from build123d import *

# Parameters (mm, degrees)
SKETCH1_R           = 1.6
BOSS_EXTRUDE1_DEPTH = 6
CUT_EXTRUDE1_DEPTH  = 2.5
SKETCH3_R           = 2.75
CUT_EXTRUDE2_DEPTH  = 3
FILLET1_R           = 2


with BuildPart() as part:
    # Sketch1 → Boss-Extrude1 (new body)
    with BuildSketch(Plane(origin=(0, 0, 0), x_dir=(1, 0, 0), z_dir=(0, 1, 0))):
        Polygon((-7.472353521, 4.877749034), (-7.472353521, -6.298721554), (7.527646479, -6.298721554), (7.527646479, 8.701278446), (-7.472353521, 8.701278446), align=None)
        with Locations(Location((-3.722353521, 4.951278446, 0), (0, 0, 270))):
            Circle(SKETCH1_R, mode=Mode.SUBTRACT)
        with Locations(Location((3.777646479, -2.548721554, 0), (0, 0, 270))):
            Circle(SKETCH1_R, mode=Mode.SUBTRACT)
        with Locations(Location((3.777646479, 4.951278446, 0), (0, 0, 270))):
            Circle(SKETCH1_R, mode=Mode.SUBTRACT)
        with Locations(Location((-3.722353521, -2.548721554, 0), (0, 0, 270))):
            Circle(SKETCH1_R, mode=Mode.SUBTRACT)
    extrude(amount=BOSS_EXTRUDE1_DEPTH)

    # Sketch2 → Cut-Extrude1 (cut)
    with BuildSketch(Plane(origin=(0, 6, 0), x_dir=(1, 0, 0), z_dir=(0, 1, 0))):
        Polygon((-2.109264929, 2.216085852), (-0.547062955, 4.980657848), (-2.160151547, 7.715850442), (-5.335442114, 7.686471039), (-6.897644088, 4.921899043), (-5.284555496, 2.186706449), align=None)
        Polygon((7.097410526, -2.548721554), (5.437528503, 0.326278446), (2.117764455, 0.326278446), (0.457882431, -2.548721554), (2.117764455, -5.423721554), (5.437528503, -5.423721554), align=None)
    extrude(amount=-CUT_EXTRUDE1_DEPTH, mode=Mode.SUBTRACT)

    # Sketch3 → Cut-Extrude2 (cut)
    with BuildSketch(Plane.XZ):
        with Locations(Location((3.777646479, -4.951278446, 0), (0, 0, 270))):
            Circle(SKETCH3_R)
        with Locations(Location((-3.722353521, 2.548721554, 0), (0, 0, 270))):
            Circle(SKETCH3_R)
    extrude(amount=-CUT_EXTRUDE2_DEPTH, mode=Mode.SUBTRACT)

    # Fillet1
    fillet1_edges = [part.edges().sort_by_distance(p)[0] for p in [
        (-7.472353521, 3, -8.701278446),
        (7.527646479, 3, -8.701278446),
        (7.527646479, 3, 6.298721554),
        (-7.472353521, 3, 6.298721554),
    ]]
    fillet(fillet1_edges, radius=FILLET1_R)


solid = part.part
Geometry: final body of the model. Coordinates: model frame, mm. A direction names the side the tool comes from. Round coordinates to 2 decimals unless told otherwise and drop trailing zeros. Loops run counter-clockwise (first coordinate to the right, second up) from the corner with the lowest first, then second, coordinate; pieces in that order, holes last.
Q1. Pull-direction query (X, two-part tool) for faces 1 (the flat face through (0, 6, -1)), 2 (the cylindrical face through (-2.373, 4.479, 3.409)), 3 (the cylindrical face through (-6.9, 3, -8.1)), 4 (the flat face through (2, 3.5, 2)); classes: released by +X, released by -X, zero draft, split by the parting line, or undercut.
Q2. Access query for faces 5 (the cylindrical face through (2.72, 1.48, -7.49)), 6 (the flat face through (1.28, 4.77, 3.97)), 7 (the flat face through (0, 0, -1)). Directions: +Z, -Z, +X, -X, +Y, -Y. A direction counts if a zero-diameter tool reaches every point of the face in a straight line with its end or side. Return the directions, or none.
Q3. Section D-D on x = 0.75. Return loops of the section in (y, z), plus the area to 3 significant figures.
Q4. Material intervals for L1, parallel to X at y = 2.4, z = 3.75; L2, parallel to X at y = 4.7, z = 3; L3, parallel to Z at x = 4.25, y = 0.6, sorted ascending.
Q5. Pin query (flat end, axial travel): P1, Ø3, axis at x = -4, z = 3.5, coming from the -Y side; P2, Ø3, axis at x = -3.72, z = 2.55, coming from the +Y side; P3, Ø3, axis at x = -3, z = -4.5, coming from the +Y side. Return the tip coordinate at first contact, or that it passes through.
Q6. Section C-C on z = -6. Return loops of the section in (x, y), plus the area to 3 significant figures.
Q7. Section B-B on y = 0.4. Return loops of the section in (x, z), plus the area to 3 significant figures.
Q8. Section A-A on x = 3. Return loops of the section in (y, z), plus the area to 3 significant figures.
Evaluation:
1. face 1: zero draft
1. face 2: undercut
1. face 3: released by -X
1. face 4: undercut
2. face 5: -Y
2. face 6: +Y
2. face 7: +Z, -Z, +X, -X, -Y
3. outline: (0, -8.7) - (6, -8.7) - (6, 2.04) - (3.5, 2.04) - (3.5, 3.05) - (6, 3.05) - (6, 6.3) - (0, 6.3) - close
3. area: 87.5 mm2
4. L1: x = -7.47 to -6.2, -1.25 to 2.72, 4.83 to 7.53
4. L2: x = -7.47 to -5.26, -2.19 to 0.72, 6.84 to 7.53
4. L3: z = -8.7 to -7.66, -2.24 to 1.02, 4.08 to 6.3
5. P1: stops at y = 3
5. P2: passes through
5. P3: stops at y = 3.5
6. outline: (-7.47, 0) - (-4.93, 0) - (-4.93, 3.5) - (-6.29, 3.5) - (-6.29, 6) - (-7.47, 6) - close; (-2.51, 0) - (1.24, 0) - (1.24, 3) - (2.57, 3) - (2.57, 6) - (-1.15, 6) - (-1.15, 3.5) - (-2.51, 3.5) - close; (4.99, 3) - (6.32, 3) - (6.32, 0) - (7.53, 0) - (7.53, 6) - (4.99, 6) - close
6. area: 46.2 mm2
7. outline: (-7.47, -6.7) arc R2 ccw to (-5.47, -8.7) - (5.53, -8.7) arc R2 ccw to (7.53, -6.7) - (7.53, 4.3) arc R2 ccw to (5.53, 6.3) - (-5.47, 6.3) arc R2 ccw to (-7.47, 4.3) - close; hole circle Ø5.5 at (-3.72, 2.55); hole circle Ø3.2 at (-3.72, -4.95); hole circle Ø5.5 at (3.78, -4.95); hole circle Ø3.2 at (3.78, 2.55)
7. area: 158 mm2
8. outline: (0, -8.7) - (6, -8.7) - (6, -6.35) - (3, -6.35) - (3, -7.59) - (0, -7.59) - close; (0, -2.31) - (3, -2.31) - (3, -3.55) - (6, -3.55) - (6, -0.33) - (3.5, -0.33) - (3.5, 1.15) - (0, 1.15) - close; (0, 3.95) - (3.5, 3.95) - (3.5, 5.42) - (6, 5.42) - (6, 6.3) - (0, 6.3) - close
8. area: 41.6 mm2
